Here's how the part is built. I have some questions about the finished solid (model axes, mm). A direction names the side the tool comes from. Coordinates: 2 decimals unless noted, no trailing zeros. Order: outer loops, then holes, each group sorted by start corner. A loop starts at its lowest first (then second) coordinate and runs counter-clockwise, first axis right, second up.
```python
from build123d import *

# Parameters (mm, degrees)
PAD_DEPTH    = 40
SKETCH001_W  = 35
SKETCH001_H  = 135
PAD001_DEPTH = 555
SKETCH002_W  = 70
SKETCH002_H  = 40
PAD002_DEPTH = 395
SKETCH003_W  = 70
SKETCH003_H  = 40
PAD003_DEPTH = 305
SKETCH004_R  = 3.125
POCKET_DEPTH = 595.001


with BuildPart() as part:
    # Sketch → Pad (new body)
    with BuildSketch(Plane.XY):
        Polygon((-560, 67.5), (560, 67.5), (560, 157.5), (595, 157.5), (595, -372.5), (560, -372.5), (560, -67.5), (-560, -67.5), (-560, -372.5), (-595, -372.5), (-595, 157.5), (-560, 157.5), align=None)
    extrude(amount=PAD_DEPTH)

    # Sketch001 (on Face14 of Pad) → Pad001 (join)
    with BuildSketch(Plane.XY.offset(40)):
        with Locations((-577.5, 0)):
            Rectangle(SKETCH001_W, SKETCH001_H)
        with Locations((577.5, 0)):
            Rectangle(SKETCH001_W, SKETCH001_H)
    extrude(amount=PAD001_DEPTH)

    # Sketch002 (on Face27 of Pad001) → Pad002 (join)
    with BuildSketch(Plane.XZ.offset(67.5)):
        with Locations((-577.5, 575)):
            Rectangle(SKETCH002_W, SKETCH002_H)
        with Locations((577.5, 575)):
            Rectangle(SKETCH002_W, SKETCH002_H)
    extrude(amount=PAD002_DEPTH)

    # Sketch003 (on Face32 of Pad002) → Pad003 (join)
    with BuildSketch(Plane(origin=(0, -67.5, 0), x_dir=(-1, 0, 0), z_dir=(0, 1, 0))):
        with Locations((577.5, 575)):
            Rectangle(SKETCH003_W, SKETCH003_H)
        with Locations((-577.5, 575)):
            Rectangle(SKETCH003_W, SKETCH003_H)
    extrude(amount=PAD003_DEPTH)

    # Sketch004 (on Face47 of Pad003) → Pocket (cut, through all)
    with BuildSketch(Plane.XY.offset(595)):
        with Locations((-577.5, -427.5)):
            Circle(SKETCH004_R)
        with Locations((577.5, -427.5)):
            Circle(SKETCH004_R)
        with Locations((-577.5, 202.5)):
            Circle(SKETCH004_R)
        with Locations((577.5, 202.5)):
            Circle(SKETCH004_R)
    extrude(amount=-POCKET_DEPTH, mode=Mode.SUBTRACT)


solid = part.part
```
Q1. For faces 1 (the flat face through (577, 67.5, 294)), 2 (the flat face through (560, 112, 20)), 3 (the flat face through (-578, -67.5, 294)), 4 (the flat face through (-595, -52, 212)), which set-ups out of +Z, -Z, +X, -X, +Y, -Y let a thin tool reach every point of the face, with its end or its side?
Q2. If we section it at D-D on y = -14: Write out the boundary of the cut face in (x, z).
Q3. If we section it at B-B on y = 93: Write out the boundary of the cut face in (x, z).
Q4. If we section it at C-C on y = -405.5: Write out the boundary of the cut face in (x, z).
Q5. If we section it at A-A on z = 472: Write out the boundary of the cut face in (x, y), then the cut area to 3 significant figures.
Q6. We'd pull the mould along X, two halves only. Please class faces 5 (the flat face through (-560, -218, 20)), 6 (the flat face through (-578, -462.5, 575)), 7 (the flat face through (595, -28, 235)): pulls with the +X half, pulls with the -X half, needs draft (parallel to the pull), parting line crosses it, or undercut.
Q7. Will these pins go through, and if not, where does the flat tip stop? pin 1 (12 mm diameter, centred on x = -47, z = 28, fed in from -Y); pin 2 (4 mm diameter, centred on y = -2.5, z = 201.5, fed in from -X); pin 3 (20 mm diameter, centred on y = 105, z = 16.5, fed in from +X).
Q8. I need wall thicknesses on L1, parallel to X at y = 202.5, z = 572.5 (3 decimals); L2, parallel to Y at x = -577.5, z = 586.5 (3 decimals); L3, parallel to Z at x = 55.5, y = 2. Which ranges of each line are inside material? Lowest first, please.
Reply:
1. face 1: +X, -X, +Y
1. face 2: -Z, +Y
1. face 3: +X, -X, -Y
1. face 4: -Z, -X, +Y, -Y
2. outline: (-612.5, 555) - (-595, 555) - (-595, 0) - (595, 0) - (595, 555) - (612.5, 555) - (612.5, 595) - (542.5, 595) - (542.5, 555) - (560, 555) - (560, 40) - (-560, 40) - (-560, 555) - (-542.5, 555) - (-542.5, 595) - (-612.5, 595) - close
3. outline: (-612.5, 555) - (-542.5, 555) - (-542.5, 595) - (-612.5, 595) - close; (-595, 0) - (-560, 0) - (-560, 40) - (-595, 40) - close; (542.5, 555) - (612.5, 555) - (612.5, 595) - (542.5, 595) - close; (560, 0) - (595, 0) - (595, 40) - (560, 40) - close
4. outline: (-612.5, 555) - (-542.5, 555) - (-542.5, 595) - (-612.5, 595) - close; (542.5, 555) - (612.5, 555) - (612.5, 595) - (542.5, 595) - close
5. outline: (-595, -67.5) - (-560, -67.5) - (-560, 67.5) - (-595, 67.5) - close; (560, -67.5) - (595, -67.5) - (595, 67.5) - (560, 67.5) - close
5. area: 9,450 mm2
6. face 5: undercut
6. face 6: needs draft
6. face 7: pulls with the +X half
7. pin 1: stops at y = -67.5
7. pin 2: stops at x = -595
7. pin 3: stops at x = 595
8. L1: x = -612.5 to -580.625, -574.375 to -542.5, 542.5 to 574.375, 580.625 to 612.5
8. L2: y = -462.5 to -430.625, -424.375 to 199.375, 205.625 to 237.5
8. L3: z = 0 to 40
